Verification items for the finished model (mm, model axes). A direction names the side the tool comes from. Coordinates: 2 decimals unless noted, no trailing zeros. Loops run counter-clockwise (first coordinate to the right, second up) from the corner with the lowest first, then second, coordinate; pieces in that order, holes last. Notation, with made-up numbers: (85, 44.25) -> (99, 44.25) arc R24 ccw to (99, 80.25) -> close; hole circle Ø5 at (74, -39). An arc over 180 degrees is marked (long way). Write item = value, one per line.
```python
from build123d import *

# Parameters (mm, degrees)
F1_DEPTH     = 13.75
F2_W         = 10
F2_H         = 5
F3_DEPTH     = 10
F4_R         = 1
F5_T1_DEPTH  = 5
F5_T4_ANGLE  = 90
F5_T6_ANGLE  = 90
F5_T8_ANGLE  = 90
F5_T10_ANGLE = 90


# Not quite as in the source:
# - a fillet or chamfer that OpenCascade refuses, or shapes differently, is made with other operations: its cross-section is extruded or revolved along the edge and cut away or added


with BuildPart() as f1:
    # F0 (on Top) → F1 (new body)
    with BuildSketch(Plane.XY):
        with BuildLine():
            Line((7.9270144597, -2.8950429987), (-17.0730578044, -2.8950429987))
            Line((-17.0730578044, -2.8950429987), (-17.0730578044, -7.8164328754))
            Line((-17.0730578044, -7.8164328754), (-17.0730578044, -10.3164328754))
            Line((-17.0730578044, -10.3164328754), (-15.0730578044, -10.3164328754))
            Line((-15.0730578044, -10.3164328754), (-15.0730578044, -7.8164328754))
            ThreePointArc((-15.0730578044, -7.8164328754), (-12.5730578044, -5.3164328754), (-10.0730578044, -7.8164328754))
            Line((-10.0730578044, -7.8164328754), (-10.0730578044, -10.3164328754))
            Line((-10.0730578044, -10.3164328754), (0.9269421956, -10.3164328754))
            Line((0.9269421956, -10.3164328754), (0.9269421956, -7.8164328754))
            ThreePointArc((0.9269421956, -7.8164328754), (3.4269421956, -5.3164328754), (5.9269421956, -7.8164328754))
            Line((5.9269421956, -7.8164328754), (5.9269421956, -10.3164328754))
            Line((5.9269421956, -10.3164328754), (7.9270144597, -10.3164328754))
            Line((7.9270144597, -10.3164328754), (7.9270144597, -7.8164328754))
            Line((7.9270144597, -7.8164328754), (7.9270144597, -2.8950429987))
        make_face()
    extrude(amount=F1_DEPTH)

    # F2 (on face) → F3 (join)
    with BuildSketch(Plane(origin=(0, -2.8950429987, 0), x_dir=(-1, 0, 0), z_dir=(0, 1, 0))):
        with Locations((4.5730578044, 6.875)):
            Rectangle(F2_W, F2_H)
    extrude(amount=F3_DEPTH)

    # F4
    f4_edges = [f1.edges().sort_by_distance(p)[0] for p in [
        (-4.573058, 7.104957, 9.375),
        (-4.573058, 7.104957, 4.375),
        (-9.573058, 2.104957, 4.375),
        (-9.573058, 2.104957, 9.375),
        (0.426942, 2.104957, 9.375),
        (0.426942, 2.104957, 4.375),
    ]]
    fillet(f4_edges, radius=F4_R)

    # F5: fillet of radius 5 on 2 edges, made by hand

    # F5_s2 → F5_t1 (cut)
    with BuildSketch(Plane.XY.offset(4.375)):
        with BuildLine():
            ThreePointArc((-9.5730578044, 2.1049570013), (-8.1085917103, 5.6404909072), (-4.5730578044, 7.1049570013))
            Line((-4.5730578044, 7.1049570013), (-9.5730578044, 7.1049570013))
            Line((-9.5730578044, 7.1049570013), (-9.5730578044, 2.1049570013))
        make_face()
        with BuildLine():
            ThreePointArc((0.4269421956, 2.1049570013), (-1.0375238985, 5.6404909072), (-4.5730578044, 7.1049570013))
            Line((-4.5730578044, 7.1049570013), (0.4269421956, 7.1049570013))
            Line((0.4269421956, 7.1049570013), (0.4269421956, 2.1049570013))
        make_face()
    extrude(amount=F5_T1_DEPTH, mode=Mode.SUBTRACT)

    # F5_s3 → F5_t4 (revolve, cut)
    with BuildSketch(Plane.XZ.offset(-2.1049570013)):
        with BuildLine():
            ThreePointArc((-0.5730578044, 9.375), (0.1340489768, 9.0821067812), (0.4269421956, 8.375))
            Line((0.4269421956, 8.375), (0.4269421956, 9.375))
            Line((0.4269421956, 9.375), (-0.5730578044, 9.375))
        make_face()
    revolve(axis=Axis((-4.5730578044, 2.1049570013, 9.375), (0, 0, 1)), revolution_arc=F5_T4_ANGLE, mode=Mode.SUBTRACT)

    # F5_s5 → F5_t6 (revolve, cut)
    with BuildSketch(Plane.YZ.offset(-4.5730578044)):
        with BuildLine():
            ThreePointArc((6.1049570013, 4.375), (6.8120637825, 4.6678932188), (7.1049570013, 5.375))
            Line((7.1049570013, 5.375), (7.1049570013, 4.375))
            Line((7.1049570013, 4.375), (6.1049570013, 4.375))
        make_face()
    revolve(axis=Axis((-4.5730578044, 2.1049570013, 4.375), (0, 0, -1)), revolution_arc=F5_T6_ANGLE, mode=Mode.SUBTRACT)

    # F5_s7 → F5_t8 (revolve, cut)
    with BuildSketch(Plane.XZ.offset(-2.1049570013)):
        with BuildLine():
            ThreePointArc((-8.5730578044, 4.375), (-9.2801645856, 4.6678932188), (-9.5730578044, 5.375))
            Line((-9.5730578044, 5.375), (-9.5730578044, 4.375))
            Line((-9.5730578044, 4.375), (-8.5730578044, 4.375))
        make_face()
    revolve(axis=Axis((-4.5730578044, 2.1049570013, 4.375), (0, 0, -1)), revolution_arc=F5_T8_ANGLE, mode=Mode.SUBTRACT)

    # F5_s9 → F5_t10 (revolve, cut)
    with BuildSketch(Plane.YZ.offset(-4.5730578044)):
        with BuildLine():
            ThreePointArc((6.1049570013, 9.375), (6.8120637825, 9.0821067812), (7.1049570013, 8.375))
            Line((7.1049570013, 8.375), (7.1049570013, 9.375))
            Line((7.1049570013, 9.375), (6.1049570013, 9.375))
        make_face()
    revolve(axis=Axis((-4.5730578044, 2.1049570013, 9.375), (0, 0, 1)), revolution_arc=F5_T10_ANGLE, mode=Mode.SUBTRACT)


solid = f1.part
```
1) Release check for a two-part mould opening along X. For faces 1 (the face through (-17.073, -7, 7)), 2 (the face through (5.927, -9, 7)), 3 (the face through (0.142, -0.36, 9.074)) record: pulls with the +X half, pulls with the -X half, needs draft (parallel to the pull), parting line crosses it, or undercut.
Ans:
face_1 = pulls with the -X half
face_2 = undercut
face_3 = pulls with the +X half
2) Sectioned sample at B-B, the plane y = 0.25. Record the cut outline in (x, z) (3 decimals), plus the area to 3 significant figures.
Ans:
outline = (-9.573, 5.375) arc R1 ccw to (-8.573, 4.375) -> (-0.573, 4.375) arc R1 ccw to (0.427, 5.375) -> (0.427, 8.375) arc R1 ccw to (-0.573, 9.375) -> (-8.573, 9.375) arc R1 ccw to (-9.573, 8.375) -> close
area = 49.1 mm2
3) Material ranges on line 1 (X direction, y = -9.5, z = 7.75); line 2 (X direction, y = -7.25, z = 13.25); line 3 (Y direction, x = -8.5, z = 10), recorded low to high.
Ans:
line_1 = -17.07 to -15.07, -10.07 to 0.93, 5.93 to 7.93
line_2 = -17.07 to -15.01, -10.14 to 0.99, 5.86 to 7.93
line_3 = -10.32 to -2.9
4) Depth check by flat-ended pin: pin 1 Ø1 at (y, z) = (4, 6.5) entering from -X; pin 2 Ø4 at (x, z) = (5.5, 10.5) entering from +Y; pin 3 Ø4 at (y, z) = (0.5, 3) entering from +X. Enter the tip coordinate at first touch or a pass-through.
Ans:
pin_1 = -9.37
pin_2 = -2.9
pin_3 = 0.35
5) Tool access check on faces 4 (the face through (-9.573, 0, 7)), 5 (the face through (-15.073, -9, 7)), 6 (the face through (-9.27, -0.36, 9.09)), 7 (the face through (0.142, -0.36, 4.676)). Record the directions out of +Z, -Z, +X, -X, +Y, -Y that give a thin tool (end or side, any length) a straight path to the whole face; none if there is none.
Ans:
face_4 = +Z, -Z, -X, +Y
face_5 = +Z, -Z, -Y
face_6 = +Z, -X, +Y
face_7 = -Z, +X, +Y
6) Sectioned sample at A-A, the plane z = 6.25. Record the cut outline in (x, y), plus the area to 3 significant figures.
Ans:
outline = (-17.07, -10.32) -> (-15.07, -10.32) -> (-15.07, -7.82) arc R2.5 cw to (-10.07, -7.82) -> (-10.07, -10.32) -> (0.93, -10.32) -> (0.93, -7.82) arc R2.5 cw to (5.93, -7.82) -> (5.93, -10.32) -> (7.93, -10.32) -> (7.93, -2.9) -> (0.43, -2.9) -> (0.43, 2.1) arc R5 ccw to (-9.57, 2.1) -> (-9.57, -2.9) -> (-17.07, -2.9) -> close
area = 230 mm2
7) Sectioned sample at D-D, the plane x = 5.25. Record the cut outline in (y, z).
Ans:
outline = (-6.11, 0) -> (-2.9, 0) -> (-2.9, 13.75) -> (-6.11, 13.75) -> close
8) Sectioned sample at C-C, the plane z = 4. Record the cut outline in (x, y), plus the area to 3 significant figures.
Ans:
outline = (-17.07, -10.32) -> (-15.07, -10.32) -> (-15.07, -7.82) arc R2.5 cw to (-10.07, -7.82) -> (-10.07, -10.32) -> (0.93, -10.32) -> (0.93, -7.82) arc R2.5 cw to (5.93, -7.82) -> (5.93, -10.32) -> (7.93, -10.32) -> (7.93, -2.9) -> (-17.07, -2.9) -> close
area = 141 mm2
